from build123d import *

# Parameters (mm, degrees)
F0_W     = 5.5
F0_H     = 8
F1_DEPTH = 5
F0_R     = 1
F2_COUNT = 4
F4_W     = 5.5
F4_H     = 8
F4_W_2   = 8
F4_H_2   = 5.5
F5_DEPTH = 10


with BuildPart() as f1:
    # F0 (on Top) → F1 (new body)
    with BuildSketch(Plane.XY):
        with Locations((0, 8)):
            Rectangle(F0_W, F0_H)
    extrude(amount=F1_DEPTH)


with BuildPart() as f1b:
    # F0 (on Top) → F1, piece 2 (new body)
    with BuildSketch(Plane.XY):
        Circle(F0_R)
    extrude(amount=F1_DEPTH)


with BuildPart() as f2_1:
    # F2: instance of F1
    add(f1.part.rotate(Axis((0, 0, 0), (0, 0, -1)), 1 * 360 / F2_COUNT))


with BuildPart() as f2_2:
    # F2: instance of F1
    add(f1.part.rotate(Axis((0, 0, 0), (0, 0, -1)), 2 * 360 / F2_COUNT))


with BuildPart() as f2_3:
    # F2: instance of F1
    add(f1.part.rotate(Axis((0, 0, 0), (0, 0, -1)), 3 * 360 / F2_COUNT))


with BuildPart() as f1_1:
    add(f1.part)

    add(f2_1.part)  # F5 merges F2_1

    add(f2_2.part)  # F5 merges F2_2

    add(f2_3.part)  # F5 merges F2_3
    # F4 (on face) → F5 (join)
    with BuildSketch(Plane.XY.offset(5)):
        with Locations((0, 8)):
            Rectangle(F4_W, F4_H)
        Polygon((12, 12), (2.75, 12), (2.75, 4), (-2.75, 4), (-2.75, 12), (-12, 12), (-12, 2.75), (-4, 2.75), (-4, -2.75), (-12, -2.75), (-12, -12), (-2.75, -12), (-2.75, -4), (2.75, -4), (2.75, -12), (12, -12), (12, -2.75), (4, -2.75), (4, 2.75), (12, 2.75), align=None)
        with Locations((8, 0)):
            Rectangle(F4_W_2, F4_H_2)
        with Locations((-8, 0)):
            Rectangle(F4_W_2, F4_H_2)
        with Locations((0, -8)):
            Rectangle(F4_W, F4_H)
    extrude(amount=F5_DEPTH)


solid = f1_1.part
Check sheet for the modelled part. Datum: model origin and axes. Units: mm. A direction names the side the tool comes from. Round coordinates to 2 decimals unless told otherwise and drop trailing zeros. Order: outer loops, then holes, each group sorted by start corner. A loop starts at its lowest first (then second) coordinate and runs counter-clockwise, first axis right, second up. Notation, with made-up numbers: M 68,45 L 114,45 A15 cw 114,53 Z; hole C 86.25,-25 d10. An arc over 180 degrees is marked long. One line per item, written item: value. Start each with the question number.
1. Gauge pin test, flat ends, axial feed: P1, Ø4, axis at x = 7.5, z = 2.5, coming from the -Y side; P2, Ø4, axis at x = -10, z = 2.5, coming from the -Y side; P3, Ø4, axis at y = -8, z = 2.5, coming from the -X side. Record the tip position at first contact, or that the pin passes through.
2. Release check for a two-part mould opening along X. For faces 1 (the flat face through (2.75, -8, 2)), 2 (the flat face through (0, -12, 9)), 3 (the flat face through (4, 0, 2)) record: released by +X, released by -X, zero draft, split by the parting line, or undercut.
3. Scan lines: line 1 along Z through (x, y) = (-8.5, 9.75); line 2 along Y through (x, z) = (-10.5, 3). Record each from-to range of solid material in increasing order.
4. Section check A-A on z = 1.75. Enter the section's corners in (x, y), and give its area (3 significant figures).
5. Section check C-C on y = -1.75. Enter the section's corners in (x, z).
6. Section check B-B on x = 8.5. Enter the section's corners in (y, z), and give its area (4 significant figures).
7. Access from +Z, -Z, +X, -X, +Y, -Y to the whole of each face (thin tool, end or side, straight path). Record for faces 4 (the flat face through (2.75, 8, 2)), 5 (the flat face through (-8, 2.75, 2)), 6 (the flat face through (-2.75, 8, 2)).
Results found:
1. P1: y = -2.75
1. P2: y = -2.75
1. P3: x = -2.75
2. face 1: released by +X
2. face 2: zero draft
2. face 3: undercut
3. line 1: 5 to 15
3. line 2: -2.75 to 2.75
4. outline: M -12,-2.75 L -4,-2.75 L -4,2.75 L -12,2.75 Z; M -2.75,-12 L 2.75,-12 L 2.75,-4 L -2.75,-4 Z; M -2.75,4 L 2.75,4 L 2.75,12 L -2.75,12 Z; M 4,-2.75 L 12,-2.75 L 12,2.75 L 4,2.75 Z
4. area: 176 mm^2
5. outline: M -12,0 L -4,0 L -4,5 L 4,5 L 4,0 L 12,0 L 12,15 L -12,15 Z
6. outline: M -12,5 L -2.75,5 L -2.75,0 L 2.75,0 L 2.75,5 L 12,5 L 12,15 L -12,15 Z
6. area: 267.5 mm^2
7. face 4: -Z, +X, +Y, -Y
7. face 5: -Z, +X, -X, +Y
7. face 6: -Z, -X, +Y, -Y
